The drawing under review shows one solid part. Ordinate dimensions are in mm from its lowest x, y, z. Coordinates: 2 decimals unless noted, no trailing zeros. Write each loop counter-clockwise with the first axis right and the second up, starting at its lowest first coordinate (ties: lowest second). Pieces come first, ordered by that corner, then holes. Notation, with made-up numbers: (22.25, 76) -> (71.25, 76) arc R26 cw to (71.25, 93) -> close; hole circle Ø10 at (-28, 77). An arc over 180 degrees is marked (long way). One line per question, with ' | ' between items. Start each with the question number.
Q1. Add section A-A on y = 150. State the section outline as (x, z) points.
Q2. Wall thickness on probe 1 along Y at (x, z) = (550, 18); probe 2 along Y at (x, z) = (330, 11.5); probe 3 along X at (y, z) = (193, 27): over which ranges is each line inside the solid? List them lowest first.
Q3. For P1, Ø1, axis at x = 98, y = 98, coming from the -Z side, flat-tipped, find the tip position at first contact; note if it passes through.
Q4. Add section C-C on x = 550. State the section outline as (y, z) points, and give its area (3 significant figures).
Q5. Draft analysis for pull direction Y (two halves, no side actions). For the marked faces 1, 2 and 3, state which applies: pulls with the +Y half, pulls with the -Y half, needs draft (parallel to the pull), parting line crosses it, or undercut.
Q6. Add section D-D on y = 94. State the section outline as (x, z) points.
Q7. Add section B-B on z = 57.5. State the section outline as (x, y) points.
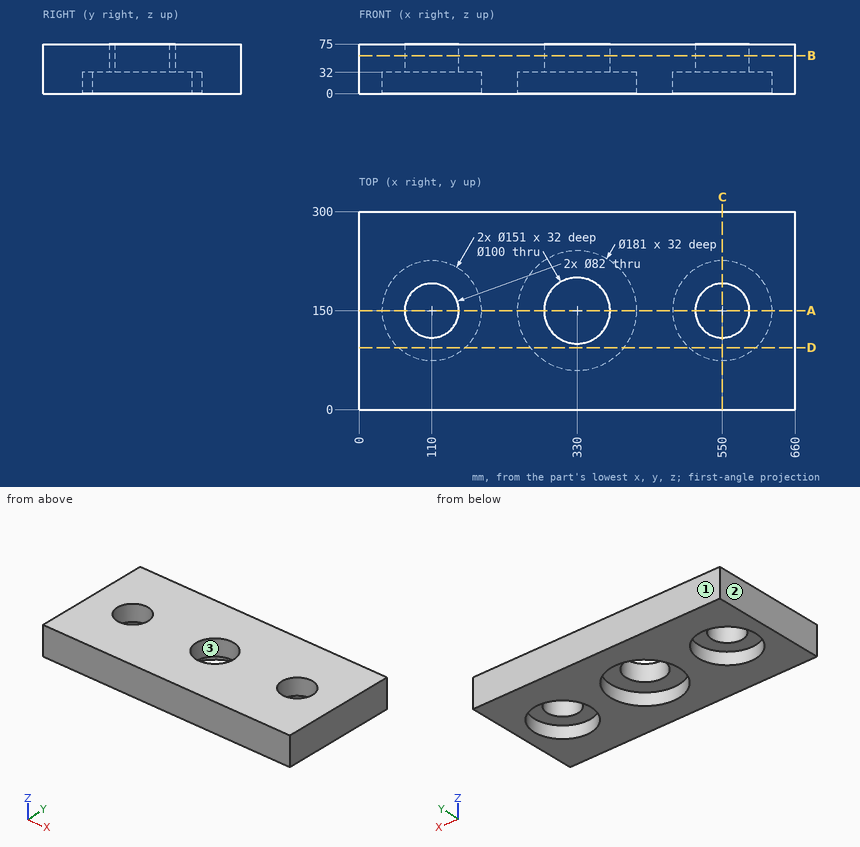
Output values:
1) outline: (0, 0) -> (34.5, 0) -> (34.5, 32) -> (69, 32) -> (69, 75) -> (0, 75) -> close; (151, 32) -> (185.5, 32) -> (185.5, 0) -> (239.5, 0) -> (239.5, 32) -> (280, 32) -> (280, 75) -> (151, 75) -> close; (380, 32) -> (420.5, 32) -> (420.5, 0) -> (474.5, 0) -> (474.5, 32) -> (509, 32) -> (509, 75) -> (380, 75) -> close; (591, 32) -> (625.5, 32) -> (625.5, 0) -> (660, 0) -> (660, 75) -> (591, 75) -> close
2) probe 1: y = 0 to 74.5, 225.5 to 300 | probe 2: y = 0 to 59.5, 240.5 to 300 | probe 3: x = 0 to 47.94, 172.06 to 250.37, 409.63 to 487.94, 612.06 to 660
3) P1: stops at z = 32
4) outline: (0, 0) -> (74.5, 0) -> (74.5, 32) -> (109, 32) -> (109, 75) -> (0, 75) -> close; (191, 32) -> (225.5, 32) -> (225.5, 0) -> (300, 0) -> (300, 75) -> (191, 75) -> close | area: 14,100 mm2
5) face 1: pulls with the +Y half | face 2: needs draft | face 3: undercut
6) outline: (0, 0) -> (59.36, 0) -> (59.36, 32) -> (160.64, 32) -> (160.64, 0) -> (258.91, 0) -> (258.91, 32) -> (401.09, 32) -> (401.09, 0) -> (499.36, 0) -> (499.36, 32) -> (600.64, 32) -> (600.64, 0) -> (660, 0) -> (660, 75) -> (0, 75) -> close
7) outline: (0, 0) -> (660, 0) -> (660, 300) -> (0, 300) -> close; hole circle Ø82 at (110, 150); hole circle Ø100 at (330, 150); hole circle Ø82 at (550, 150)
